Autodesk Inventor part; units mm, degrees
ref_plane "YZ Plane" through (0, 0, 0) normal (1, 0, 0) x (0, 1, 0)
ref_plane "XZ Plane" through (0, 0, 0) normal (0, 1, 0) x (-1, 0, 0)
ref_plane "XY Plane" through (0, 0, 0) normal (0, 0, 1) x (1, 0, 0)
sketch "Sketch1" plane through (0, 0, 0) normal (0, 0, 1) x (1, 0, 0)
  circle A0 centre (0, 0) radius 7
  line L0 (-4.95, 4.9495) -> (4.95, 4.9495)
  line L1 (-4.95, -4.9495) -> (4.95, -4.9495)
  line L2 (0, 0) -> (0, -30) construction
  line L3 (-75, -30) -> (75, -30)
  line L4 (75, -30) -> (75, -20)
  line L5 (75, -20) -> (-75, -20)
  line L6 (-75, -20) -> (-75, -30)
  line L7 (-75, -30) -> (75, -20) construction
  line L8 (75, -30) -> (-75, -20) construction
  line L9 (-50, -20) -> (50, -20)
  line L10 (50, -20) -> (50, 30)
  line L11 (50, 30) -> (-50, 30)
  line L12 (-50, 30) -> (-50, -20)
  point P0 (0, -25)
  dimension "d1" = 7
  dimension "d2" = 9.9
  dimension "d4" = 150
  dimension "d5" = 10
  dimension "d6" = 50
  dimension "d26" = 25
  dimension "d27" = 100
  dimension "d28" = 50
extrude "Extrusion1" add sketch "Sketch1" along normal blind 28 contours L0 A0 | A0 L1 | L6 L5 L4 L3 | L12 L11 L10 L5
sketch "Sketch2" plane through (0, 0, 28) normal (0, 0, 1) x (1, 0, 0)
  line L0 (-50, -20) -> (-75, -20)
  line L1 (-75, -20) -> (-75, -30)
  line L2 (-75, -30) -> (75, -30)
  line L3 (75, -30) -> (75, -20)
  line L4 (-50, -20) -> (50, -20)
  line L5 (75, -20) -> (50, -20)
  line L6 (50, -20) -> (50, 30)
  line L7 (50, 30) -> (-50, 30)
  line L8 (-50, 30) -> (-50, -20)
  point P0 (0, 0)
extrude "Extrusion2" add sketch "Sketch2" along normal blind 32 contours L4 L5 L3 L2 L1 L0
sketch "Sketch3" plane through (0, 0, 60) normal (0, 0, 1) x (1, 0, 0)
  circle A0 centre (0, 0) radius 16
  dimension "d11" = 32
extrude "Extrusion3" cut sketch "Sketch3" against normal blind 38
sketch "Sketch4" plane through (-75, -20, 0) normal (0, 1, 0) x (1, 0, 0)
  circle A0 centre (12.5, -15) radius 3.05
  line L0 (150, 0) -> (0, 0)
  circle A1 centre (12.5, -45) radius 3.05
  circle A2 centre (47.5, -45) radius 3.05
  line L1 (75, 12) -> (75, -72)
  circle A3 centre (137.5, -15) radius 3.05
  circle A4 centre (137.5, -45) radius 3.05
  circle A5 centre (102.5, -45) radius 3.05
  line L2 (0, 0) -> (0, -60)
  point P0 (75, 0)
  point P1 (25, 0)
  point P2 (12.5, 0)
  point P3 (12.5, 0)
  point P4 (12.5, 0)
  point P5 (12.5, 0)
  dimension "d14" = 6.1
  dimension "d15" = 15
  dimension "d17" = 30
  dimension "d18" = 35
extrude "Extrusion4" cut sketch "Sketch4" against normal through all
fillet "Fillet1" radius 5 4 edges at (75, -25, 60) (-75, -25, 60) (75, -25, 0) (-75, -25, 0)
sketch "Sketch5" plane through (-50, -20, 28) normal (0, 1, 0) x (1, 0, 0)
  arc A0 (-20, 28) -> (-25, 23) centre (-20, 23) ccw
  line L0 (-25, 23) -> (-25, -27)
  line L1 (0, 28) -> (-20, 28)
  circle A1 centre (-12.5, 13) radius 3.05
  circle A2 centre (112.5, 13) radius 3.05
  arc A3 (125, 23) -> (120, 28) centre (120, 23) ccw
  line L2 (125, 23) -> (125, -27)
  circle A4 centre (-12.5, 13) radius 5.5
  circle A5 centre (-12.5, -17) radius 5.5
  circle A6 centre (22.5, -17) radius 5.5
  circle A7 centre (77.5, -17) radius 5.5
  circle A8 centre (112.5, -17) radius 5.5
  circle A9 centre (112.5, 13) radius 5.5
  arc A10 (-20, 28) -> (-25, 23) centre (-20, 23) ccw
  line L3 (-25, 23) -> (-25, -27)
  arc A11 (-25, -27) -> (-20, -32) centre (-20, -27) ccw
  line L4 (120, -32) -> (-20, -32)
  arc A12 (120, -32) -> (125, -27) centre (120, -27) ccw
  arc A13 (-25, -27) -> (-20, -32) centre (-20, -27) ccw
  line L5 (120, -32) -> (-20, -32)
  arc A14 (120, -32) -> (125, -27) centre (120, -27) ccw
  line L6 (125, 23) -> (125, -27)
  arc A15 (125, 23) -> (120, 28) centre (120, 23) ccw
  circle A16 centre (-12.5, -17) radius 3.05
  circle A17 centre (22.5, -17) radius 3.05
  circle A18 centre (77.5, -17) radius 3.05
  circle A19 centre (112.5, -17) radius 3.05
  line L7 (0, 28) -> (0, 0)
  line L8 (0, 28) -> (-20, 28)
  line L9 (120, 28) -> (100, 28)
  line L10 (100, 28) -> (100, 0)
  line L11 (0, 28) -> (0, 0)
  line L12 (120, 28) -> (100, 28)
  line L13 (100, 28) -> (100, 0)
  line L14 (0, 0) -> (100, 0)
  line L15 (0, 0) -> (100, 0)
  point P0 (50, 28)
  dimension "d22" = 11
extrude "Extrusion5" cut sketch "Sketch5" against normal blind 2 contours A1 | A2 | A4 | A5 | A6 | A7 | A8 | A9 | A16 | A17 | A18 | A19
properties part number "motor_bracket" material "Aluminum 6061"
Here's how the part is built. I have some questions about the finished solid (model axes, mm). A direction names the side the tool comes from. Coordinates: 2 decimals unless noted, no trailing zeros. Loops run counter-clockwise (first coordinate to the right, second up) from the corner with the lowest first, then second, coordinate; pieces in that order, holes last. Notation, with made-up numbers: (74, 84.5) - (133, 84.5) arc R25 cw to (133, 96.5) - close; hole circle Ø4 at (83, 77.25). An arc over 180 degrees is marked (long way). Return JSON: item names as keys, results as strings. Group by question number.
Item 1: I need wall thicknesses on line 1 (Z direction, x = 62.5, y = -21.35); line 2 (X direction, y = -24, z = 45); line 3 (Z direction, x = 27.5, y = -20.7). Which ranges of each line are inside material? Lowest first, please. Write a range as from..to.
Item 2: We'd pull the mould along Y, two halves only. Please class faces 5 (the face through (-3.47, -15.62, 25.04)), 6 (the face through (1, 30, 14)), 7 (the face through (7, 0, 11)), 8 (the face through (-68, -21, 45)): +Y half, -Y half, draft (parallel to the pull), parting line (faces both ways), or undercut.
Item 3: If we section it at B-B on x = 0: Write out the boundary of the cut face in (y, z).
Item 4: Will these pins go through, and if not, where does the flat tip stop? P1, Ø22.5, axis at y = 1, z = 15, coming from the -X side; P2, Ø12, axis at x = -62, z = 17.5, coming from the +Y side; P3, Ø12, axis at y = -4, z = 39.5, coming from the -X side; P4, Ø5, axis at x = 48, y = -20, coming from the -Z side.
Item 5: If we section it at C-C on y = -26: Write out the boundary of the cut face in (x, z), and give its area (3 significant figures).
Item 6: On a 3-axis mill with a long thin cutter (end or side, diameter ignored), from which of +Z, -Z, +X, -X, +Y, -Y can I reach the whole of each face in a straight line? I mean faces 1 (the face through (-1, -30, 30)), 2 (the face through (-60, -22, 17)), 3 (the face through (-0.7, 16.5, 28)), 4 (the face through (0, -4.95, 11)). Say none if no direction works.
Item 7: If we section it at D-D on x = 62.5: Write out the boundary of the cut face in (y, z).
Item 8: If we section it at A-A on z = 15: Write out the boundary of the cut face in (x, y).
Calculated:
{
 "1": {"line 1": "z = 0..9.5, 20.5..39.5, 50.5..60", "line 2": "x = -75..-65.55, -59.45..-30.55, -24.45..24.45, 30.55..59.45, 65.55..75", "line 3": "z = 0..39.5, 50.5..60"},
 "2": {"face 5": "undercut", "face 6": "+Y half", "face 7": "undercut", "face 8": "draft"},
 "3": {"outline": "(-30, 0) - (-4.95, 0) - (-4.95, 22) - (-16, 22) - (-16, 28) - (-20, 28) - (-20, 60) - (-30, 60) - close; (4.95, 0) - (30, 0) - (30, 28) - (16, 28) - (16, 22) - (4.95, 22) - close"},
 "4": {"P1": "stops at x = -50", "P2": "stops at y = -20", "P3": "passes through", "P4": "stops at z = 0"},
 "5": {"outline": "(-75, 5) arc R5 ccw to (-70, 0) - (70, 0) arc R5 ccw to (75, 5) - (75, 55) arc R5 ccw to (70, 60) - (-70, 60) arc R5 ccw to (-75, 55) - close; hole circle Ø6.1 at (-62.5, 15); hole circle Ø6.1 at (-62.5, 45); hole circle Ø6.1 at (-27.5, 45); hole circle Ø6.1 at (27.5, 45); hole circle Ø6.1 at (62.5, 15); hole circle Ø6.1 at (62.5, 45)", "area": "8,800 mm^2"},
 "6": {"face 1": "+Z, -Z, +X, -X, -Y", "face 2": "+Y", "face 3": "+Z, +X, -X, +Y", "face 4": "+Z, -Z"},
 "7": {"outline": "(-30, 0) - (-20, 0) - (-20, 9.5) - (-22, 9.5) - (-22, 11.95) - (-30, 11.95) - close; (-30, 18.05) - (-22, 18.05) - (-22, 20.5) - (-20, 20.5) - (-20, 39.5) - (-22, 39.5) - (-22, 41.95) - (-30, 41.95) - close; (-30, 48.05) - (-22, 48.05) - (-22, 50.5) - (-20, 50.5) - (-20, 60) - (-30, 60) - close"},
 "8": {"outline": "(-75, -30) - (-65.55, -30) - (-65.55, -22) - (-68, -22) - (-68, -20) - (-75, -20) - close; (-59.45, -30) - (59.45, -30) - (59.45, -22) - (57, -22) - (57, -20) - (50, -20) - (50, 30) - (-50, 30) - (-50, -20) - (-57, -20) - (-57, -22) - (-59.45, -22) - close; (65.55, -30) - (75, -30) - (75, -20) - (68, -20) - (68, -22) - (65.55, -22) - close; hole (-4.95, -4.95) - (4.95, -4.95) arc R7 ccw to (4.95, 4.95) - (-4.95, 4.95) arc R7 ccw to start"}
}
